```python
from build123d import *

# Parameters (mm, degrees)
CYLINDER099_R               = 3
CYLINDER099_DEPTH           = 3
CYLINDER098_R               = 5
CYLINDER098_DEPTH           = 3
CYLINDER090_R               = 1.2
CYLINDER090_DEPTH           = 13
CYLINDER091_R               = 1
CYLINDER091_DEPTH           = 12
CYLINDER091_ROLL_ANGLE      = 89.999919
CYLINDER091_PITCH_ANGLE     = -3.6e-05
CYLINDER091_PLACEMENT_ANGLE = 179.999964
CYLINDER069_R               = 2.2
CYLINDER069_DEPTH           = 12
CYLINDER069_ROLL_ANGLE      = 89.999919
CYLINDER069_PITCH_ANGLE     = -3.6e-05
CYLINDER069_PLACEMENT_ANGLE = 179.999964
CYLINDER068_R               = 1.2
CYLINDER068_DEPTH           = 12
CYLINDER068_ROLL_ANGLE      = 89.999919
CYLINDER068_PITCH_ANGLE     = -3.6e-05
CYLINDER068_PLACEMENT_ANGLE = 179.999964
BOX406016_W                 = 49
BOX406016_H                 = 2
BOX406016_DEPTH             = 32
BOX406008016_W              = 9
BOX406008016_H              = 12
BOX406008016_DEPTH          = 15
BOX406017_W                 = 16
BOX406017_H                 = 10.5
BOX406017_DEPTH             = 28
CYLINDER067_R               = 6.25
CYLINDER067_DEPTH           = 26
COMMON004_PLACEMENT_ANGLE   = 90
BOX406008015_W              = 15
BOX406008015_H              = 31
BOX406008015_DEPTH          = 15
BOX406008017_W              = 15
BOX406008017_H              = 4
BOX406008017_DEPTH          = 24
CYLINDER096_R               = 1.7
CYLINDER096_DEPTH           = 21
BOX_W                       = 15
BOX_H                       = 3
BOX_DEPTH                   = 8
CYLINDER097_R               = 1.7
CYLINDER097_DEPTH           = 21
BOX406008018_W              = 15
BOX406008018_H              = 3
BOX406008018_DEPTH          = 8
CHAMFER005_SIZE             = 1
CYLINDER093_R               = 1.7
CYLINDER093_DEPTH           = 21
CYLINDER092_R               = 1.7
CYLINDER092_DEPTH           = 21
BOX406008014_W              = 15
BOX406008014_H              = 3
BOX406008014_DEPTH          = 63
CHAMFER006_SIZE             = 1
CHAMFER007_SIZE             = 6.5


with BuildPart() as cylinder099:
    # Cylinder099 → Cylinder099 (new body)
    with BuildSketch(Plane(origin=(-9, -9, 36), x_dir=(1, 0, 0), z_dir=(0, 0, 1))):
        Circle(CYLINDER099_R)
    extrude(amount=CYLINDER099_DEPTH)


with BuildPart() as cut081:
    # Cylinder098 → Cylinder098 (new body)
    with BuildSketch(Plane(origin=(-9, -9, 36), x_dir=(1, 0, 0), z_dir=(0, 0, 1))):
        Circle(CYLINDER098_R)
    extrude(amount=CYLINDER098_DEPTH)

    # Cut081: cut Cylinder099
    add(cylinder099.part, mode=Mode.SUBTRACT)


with BuildPart() as cylinder084:
    # Cylinder090 → Cylinder090 (new body)
    with BuildSketch(Plane(origin=(0, 16, 35.8), x_dir=(1, 0, 0), z_dir=(0, -1, 0))):
        Circle(CYLINDER090_R)
    extrude(amount=CYLINDER090_DEPTH)


with BuildPart() as cylinder091:
    # Cylinder091 → Cylinder091 (new body)
    with BuildSketch(Plane.XY):
        Circle(CYLINDER091_R)
    extrude(amount=CYLINDER091_DEPTH)


with BuildPart() as cylinder091_1:
    # Cylinder091 roll: moved
    add(cylinder091.part.rotate(Axis((0, 0, 0), (1, 0, 0)), CYLINDER091_ROLL_ANGLE))


with BuildPart() as cylinder091_2:
    # Cylinder091 pitch: moved
    add(cylinder091_1.part.rotate(Axis((0, 0, 0), (0, 1, 0)), CYLINDER091_PITCH_ANGLE))


with BuildPart() as cylinder091_3:
    # Cylinder091 placement: moved
    add(cylinder091_2.part.moved(Location((11.75, -12, 42.5))).rotate(Axis((11.75, -12, 42.5), (0, 0, 1)), CYLINDER091_PLACEMENT_ANGLE))


with BuildPart() as cylinder069:
    # Cylinder069 → Cylinder069 (new body)
    with BuildSketch(Plane.XY):
        Circle(CYLINDER069_R)
    extrude(amount=CYLINDER069_DEPTH)


with BuildPart() as cylinder069_1:
    # Cylinder069 roll: moved
    add(cylinder069.part.rotate(Axis((0, 0, 0), (1, 0, 0)), CYLINDER069_ROLL_ANGLE))


with BuildPart() as cylinder069_2:
    # Cylinder069 pitch: moved
    add(cylinder069_1.part.rotate(Axis((0, 0, 0), (0, 1, 0)), CYLINDER069_PITCH_ANGLE))


with BuildPart() as cylinder069_3:
    # Cylinder069 placement: moved
    add(cylinder069_2.part.moved(Location((11.75, 3, 42.5))).rotate(Axis((11.75, 3, 42.5), (0, 0, 1)), CYLINDER069_PLACEMENT_ANGLE))


with BuildPart() as fusion103077013004017011:
    # Cylinder068 → Cylinder068 (new body)
    with BuildSketch(Plane.XY):
        Circle(CYLINDER068_R)
    extrude(amount=CYLINDER068_DEPTH)


with BuildPart() as fusion103077013004017011_1:
    # Cylinder068 roll: moved
    add(fusion103077013004017011.part.rotate(Axis((0, 0, 0), (1, 0, 0)), CYLINDER068_ROLL_ANGLE))


with BuildPart() as fusion103077013004017011_2:
    # Cylinder068 pitch: moved
    add(fusion103077013004017011_1.part.rotate(Axis((0, 0, 0), (0, 1, 0)), CYLINDER068_PITCH_ANGLE))


with BuildPart() as fusion103077013004017011_3:
    # Cylinder068 placement: moved
    add(fusion103077013004017011_2.part.moved(Location((11.75, 0, 42.5))).rotate(Axis((11.75, 0, 42.5), (0, 0, 1)), CYLINDER068_PLACEMENT_ANGLE))

    # Fusion103077013: union Cylinder069
    add(cylinder069_3.part)

    # Fusion103077013004017011: union Cylinder091
    add(cylinder091_3.part)


with BuildPart() as clamp_slot:
    # Box406016 → Box406016 (new body)
    with BuildSketch(Plane(origin=(48.48, 1, 22), x_dir=(-1, 0, 0), z_dir=(0, 0, 1))):
        with Locations((24.5, 1)):
            Rectangle(BOX406016_W, BOX406016_H)
    extrude(amount=BOX406016_DEPTH)


with BuildPart() as cube351:
    # Box406008016 → Box406008016 (new body)
    with BuildSketch(Plane(origin=(7, -6, 35), x_dir=(1, 0, 0), z_dir=(0, 0, 1))):
        with Locations((4.5, 6)):
            Rectangle(BOX406008016_W, BOX406008016_H)
    extrude(amount=BOX406008016_DEPTH)


with BuildPart() as gearbox001:
    # Box406017 → Box406017 (new body)
    with BuildSketch(Plane(origin=(-8, -5.25, 18), x_dir=(1, 0, 0), z_dir=(0, 0, 1))):
        with Locations((8, 5.25)):
            Rectangle(BOX406017_W, BOX406017_H)
    extrude(amount=BOX406017_DEPTH)


with BuildPart() as motor_hole:
    # Cylinder067 → Cylinder067 (new body)
    with BuildSketch(Plane.XY.offset(20)):
        Circle(CYLINDER067_R)
    extrude(amount=CYLINDER067_DEPTH)

    # Common004: intersect gearbox001
    add(gearbox001.part, mode=Mode.INTERSECT)


with BuildPart() as motor_hole_1:
    # Common004 placement: moved
    add(motor_hole.part.moved(Location((0, 0, 5))).rotate(Axis((0, 0, 5), (0, 0, 1)), COMMON004_PLACEMENT_ANGLE))


with BuildPart() as cut075:
    # Box406008015 → Box406008015 (new body)
    with BuildSketch(Plane(origin=(-7.5, -22, 35), x_dir=(1, 0, 0), z_dir=(0, 0, 1))):
        with Locations((7.5, 15.5)):
            Rectangle(BOX406008015_W, BOX406008015_H)
    extrude(amount=BOX406008015_DEPTH)

    # Cut073: cut motor-hole
    add(motor_hole_1.part, mode=Mode.SUBTRACT)

    # Fusion103077013004017010: union Cube351
    add(cube351.part)

    # Cut074: cut clamp-slot
    add(clamp_slot.part, mode=Mode.SUBTRACT)

    # Cut075: cut Fusion103077013004017011
    add(fusion103077013004017011_3.part, mode=Mode.SUBTRACT)


with BuildPart() as cut082:
    # Box406008017 → Box406008017 (new body)
    with BuildSketch(Plane(origin=(-7.5, 7, 26), x_dir=(1, 0, 0), z_dir=(0, 0, 1))):
        with Locations((7.5, 2)):
            Rectangle(BOX406008017_W, BOX406008017_H)
    extrude(amount=BOX406008017_DEPTH)

    # Fusion103077013004017012: union Cut075
    add(cut075.part)

    # Cut076: cut Cylinder084
    add(cylinder084.part, mode=Mode.SUBTRACT)


with BuildPart() as cut082_1:
    # Cut076 placement: moved
    add(cut082.part.moved(Location((0, 0, -5))))

    # Cut082: cut Cut081
    add(cut081.part, mode=Mode.SUBTRACT)


with BuildPart() as cylinder096:
    # Cylinder096 → Cylinder096 (new body)
    with BuildSketch(Plane(origin=(0, -13, 49), x_dir=(1, 0, 0), z_dir=(0, -1, 0))):
        Circle(CYLINDER096_R)
    extrude(amount=CYLINDER096_DEPTH)


with BuildPart() as cut080:
    # Box → Box (new body)
    with BuildSketch(Plane(origin=(-7.5, -25, 45), x_dir=(1, 0, 0), z_dir=(0, 0, 1))):
        with Locations((7.5, 1.5)):
            Rectangle(BOX_W, BOX_H)
    extrude(amount=BOX_DEPTH)

    # Cut080: cut Cylinder096
    add(cylinder096.part, mode=Mode.SUBTRACT)


with BuildPart() as cylinder097:
    # Cylinder097 → Cylinder097 (new body)
    with BuildSketch(Plane(origin=(0, -13, -22), x_dir=(1, 0, 0), z_dir=(0, -1, 0))):
        Circle(CYLINDER097_R)
    extrude(amount=CYLINDER097_DEPTH)


with BuildPart() as chamfer005:
    # Box406008018 → Box406008018 (new body)
    with BuildSketch(Plane(origin=(-7.5, -25, -26), x_dir=(1, 0, 0), z_dir=(0, 0, 1))):
        with Locations((7.5, 1.5)):
            Rectangle(BOX406008018_W, BOX406008018_H)
    extrude(amount=BOX406008018_DEPTH)

    # Cut079: cut Cylinder097
    add(cylinder097.part, mode=Mode.SUBTRACT)

    # Fusion103077013004017015: union Cut080
    add(cut080.part)

    # Chamfer005
    chamfer005_edges = [chamfer005.edges().sort_by_distance(p)[0] for p in [
        (-1.7, -22, -22),
        (-1.7, -22, 49),
    ]]
    chamfer(chamfer005_edges, length=CHAMFER005_SIZE)


with BuildPart() as cylinder093:
    # Cylinder093 → Cylinder093 (new body)
    with BuildSketch(Plane(origin=(3, -13, -4), x_dir=(1, 0, 0), z_dir=(0, -1, 0))):
        Circle(CYLINDER093_R)
    extrude(amount=CYLINDER093_DEPTH)


with BuildPart() as fusion103077013004017013:
    # Cylinder092 → Cylinder092 (new body)
    with BuildSketch(Plane(origin=(-3, -13, -14), x_dir=(1, 0, 0), z_dir=(0, -1, 0))):
        Circle(CYLINDER092_R)
    extrude(amount=CYLINDER092_DEPTH)

    # Fusion103077013004017013: union Cylinder093
    add(cylinder093.part)


with BuildPart() as fusion103077013004017017:
    # Box406008014 → Box406008014 (new body)
    with BuildSketch(Plane(origin=(-7.5, -25, -18), x_dir=(1, 0, 0), z_dir=(0, 0, 1))):
        with Locations((7.5, 1.5)):
            Rectangle(BOX406008014_W, BOX406008014_H)
    extrude(amount=BOX406008014_DEPTH)

    # Cut077: cut Fusion103077013004017013
    add(fusion103077013004017013.part, mode=Mode.SUBTRACT)

    # Chamfer006
    chamfer006_edges = [fusion103077013004017017.edges().sort_by_distance(p)[0] for p in [
        (-4.7, -25, -14),
        (1.3, -25, -4),
    ]]
    chamfer(chamfer006_edges, length=CHAMFER006_SIZE)

    # Fusion103077013004017016: union Chamfer005
    add(chamfer005.part)

    # Chamfer007
    chamfer007_edges = [fusion103077013004017017.edges().sort_by_distance(p)[0] for p in [
        (-7.5, -23.5, -26),
        (7.5, -23.5, -26),
        (7.5, -23.5, 53),
        (-7.5, -23.5, 53),
    ]]
    chamfer(chamfer007_edges, length=CHAMFER007_SIZE)

    # Fusion103077013004017017: union Cut082
    add(cut082_1.part)


solid = fusion103077013004017017.part
```
Design review of the part built by this model. Coordinates are the model's own, in mm. A direction names the side the tool comes from. Give positions to 0.01 mm unless a question says otherwise; leave off trailing zeros. Loops run counter-clockwise (first coordinate to the right, second up) from the corner with the lowest first, then second, coordinate; pieces in that order, holes last. Notation, with made-up numbers: M 3,18.25 L 18,18.25 A28 ccw 18,41.25 Z; hole C 78,-3 d7. An arc over 180 degrees is marked long. Return JSON: item names as keys, results as strings. Group by question number.
Item 1: Mouldability with a two-part tool opening along X and no side actions: class faces 4 (the flat face through (-7.5, -11.1, 30.5)), 5 (the flat face through (10, 1, 37)), 6 (the cylindrical face through (0, 9, 32)) as released by +X, released by -X, zero draft, split by the parting line, or undercut.
Item 2: We need section A-A (z = -14). Give the boundary of the cut face in (x, y).
Item 3: We need section C-C (y = -15). Give the boundary of the cut face in (x, z).
Item 4: Tool access review of faces 1 (the flat face through (5.25, -2, 37)), 2 (the cylindrical face through (-6, -9, 37)), 3 (the flat face through (0, -22, 2)): name each direction out of +Z, -Z, +X, -X, +Y, -Y from which nothing blocks a thin tool from reaching the whole face with its end or side.
Item 5: We need section D-D (x = 11.5). Give the number of separate pieces and of enclosed holes in the cut face, and give its area (3 significant figures).
Item 6: For probe 1 along X at (y, z) = (-2.6, 37.5); probe 2 along X at (y, z) = (7.7, 30.8); probe 3 along Z at (x, y) = (11.75, 2.55), list the stretches that pass through material, from the lowest coordinate up.
Item 7: We need section B-B (z = -22). Give the boundary of the cut face in (x, y).
Item 8: Insertion check: pin 1 Ø4 at (x, y) = (5, -17) entering from +Z; pin 2 Ø1.5 at (y, z) = (9.5, 35) entering from +X; pin 3 Ø3 at (x, y) = (9.5, 4) entering from -Z. Each pin has a flat end and moves straight along its axis. Give the tip position at first contact, or say it passes through.
Output:
{
 "1": {"face 4": "released by -X", "face 5": "zero draft", "face 6": "undercut"},
 "2": {"outline": "M -7.5,-25 L -5.7,-25 L -4.7,-24 L -4.7,-22 L -7.5,-22 Z; M -1.3,-24 L -0.3,-25 L 7.5,-25 L 7.5,-22 L -1.3,-22 Z"},
 "3": {"outline": "M -7.5,30 L 7.5,30 L 7.5,45 L -7.5,45 Z"},
 "4": {"face 1": "+Z, -Z", "face 2": "none", "face 3": "-Z, +X, -X"},
 "5": {"separate pieces": "4", "enclosed holes": "0", "area": "123 mm^2"},
 "6": {"probe 1": "x = -7.5 to -5.25, 5.25 to 10.75, 12.75 to 16", "probe 2": "x = -7.5 to -1.2, 1.2 to 7.5", "probe 3": "z = 30 to 36.3, 38.7 to 45"},
 "7": {"outline": "M -5,-25 L -1.7,-25 L -1.7,-23 L -2.7,-22 L -5,-22 Z; M 1.7,-25 L 5,-25 L 5,-22 L 2.7,-22 L 1.7,-23 Z"},
 "8": {"pin 1": "stops at z = 45", "pin 2": "stops at x = 7.5", "pin 3": "stops at z = 30"}
}
